```python
from build123d import *

# Parameters (mm, degrees)
SKETCH_1_R      = 77
SKETCH_1_R_2    = 75.75
EXTRUDE_1_DEPTH = 8
EXTRUDE_2_DEPTH = 3.9


with BuildPart() as part:
    # 草图1 → 凸台-拉伸1 (new body)
    with BuildSketch(Plane(origin=(0, 0, 0), x_dir=(1, 0, 0), z_dir=(0, 1, 0))):
        with Locations(Location((0, 0, 0), (0, 0, 270))):
            Circle(SKETCH_1_R)
        with Locations(Location((0, 0, 0), (0, 0, 270))):
            Circle(SKETCH_1_R_2, mode=Mode.SUBTRACT)
    extrude(amount=EXTRUDE_1_DEPTH)

    # 草图2 → 凸台-拉伸2 (add)
    with BuildSketch(Plane(origin=(0, 0, 0), x_dir=(1, 0, 0), z_dir=(0, 1, 0))):
        with BuildLine():
            Line((0, 75.75), (0, 74.85))
            ThreePointArc((0, 74.85), (27.43261682, 69.641754963), (51.047577251, 54.741824566))
            Line((51.047577251, 54.741824566), (51.661375775, 55.400042898))
            ThreePointArc((51.661375775, 55.400042898), (27.762467924, 70.479130775), (0, 75.75))
        make_face()
        with BuildLine():
            Line((55.400042898, -51.661375775), (54.741824566, -51.047577251))
            ThreePointArc((54.741824566, -51.047577251), (69.641754963, -27.43261682), (74.85, 0))
            Line((74.85, 0), (75.75, 0))
            ThreePointArc((75.75, 0), (70.479130775, -27.762467924), (55.400042898, -51.661375775))
        make_face()
        with BuildLine():
            Line((-51.661375775, -55.400042898), (-51.047577251, -54.741824566))
            ThreePointArc((-51.047577251, -54.741824566), (-27.43261682, -69.641754963), (0, -74.85))
            Line((0, -74.85), (0, -75.75))
            ThreePointArc((0, -75.75), (-27.762467924, -70.479130775), (-51.661375775, -55.400042898))
        make_face()
        with BuildLine():
            Line((-55.400042898, 51.661375775), (-54.741824566, 51.047577251))
            ThreePointArc((-54.741824566, 51.047577251), (-69.641754963, 27.43261682), (-74.85, 0))
            Line((-74.85, 0), (-75.75, 0))
            ThreePointArc((-75.75, 0), (-70.479130775, 27.762467924), (-55.400042898, 51.661375775))
        make_face()
    extrude(amount=EXTRUDE_2_DEPTH)


solid = part.part
```
Source: CAD feature listing. Evaluate the final solid. Frame: model axes, mm. A direction names the side the tool comes from. Coordinates: 2 decimals unless noted, no trailing zeros. Order: outer loops, then holes, each group sorted by start corner. A loop starts at its lowest first (then second) coordinate and runs counter-clockwise, first axis right, second up. Notation, with made-up numbers: M 36.5,-20 L 75.5,-20 A22 cw 75.5,9 Z; hole C -15,12 d2. An arc over 180 degrees is marked long. Write each question's results on one line, items separated by ' | '. Start each with the question number.
1) Section query B-B (x = -47.5). Return the cut outline in (y, z), plus the area to 3 significant figures.
2) Access query for faces 1 (the face through (-29.013, 4.833, 69.974)), 2 (the face through (-51, 8, 57)), 3 (the face through (27.066, 1.923, -69.785)). Directions: +Z, -Z, +X, -X, +Y, -Y. A direction counts if a zero-diameter tool reaches every point of the face in a straight line with its end or side. Return the directions, or none.
3) Line query: line 1 (Z direction, x = -1, y = 2.75); line 2 (X direction, y = 5, z = 0); line 3 (X direction, y = 7, z = -14). Output: solid intervals per line, ascending. Write a range as from..to.
4) Draft query along X for faces 4 (the face through (-75.17, 3.94, -16.69)), 5 (the face through (-17, 0, 74)), 6 (the face through (69.497, 1.923, 27.798)). Return one class per face: released by +X, released by -X, zero draft, split by the parting line, or undercut.
5) Section query C-C (z = -5). Return the cut outline in (x, y), plus the area to 3 significant figures.
6) Contact query for flat-ended pins moving along their axis: pin 1 Ø2 at (x, y) = (42.5, 5) entering from -Z; pin 2 Ø4 at (y, z) = (2, 4) entering from -X; pin 3 Ø3 at (x, y) = (-49, 4.5) entering from -Z; pin 4 Ø6.5 at (x, z) = (26, -66) entering from +Y. Output: stop coordinate, or through.
7) Section query A-A (y = 2.5). Return the cut outline in (x, z), plus the area to 3 significant figures.
Answers:
1) outline: M 0,-60.6 L 8,-60.6 L 8,-59.01 L 0,-59.01 Z; M 0,57.85 L 3.9,57.85 L 3.9,59.01 L 8,59.01 L 8,60.6 L 0,60.6 Z | area: 30.1 mm^2
2) face 1: +Y | face 2: +Z, -Z, +X, -X, +Y | face 3: +Y, -Y
3) line 1: z = -76.99..-75.74, 74.84..76.99 | line 2: x = -77..-75.75, 75.75..77 | line 3: x = -75.72..-74.45, 74.45..75.72
4) face 4: split by the parting line | face 5: zero draft | face 6: undercut
5) outline: M -76.84,0 L -74.68,0 L -74.68,3.9 L -75.58,3.9 L -75.58,8 L -76.84,8 Z; M 75.58,0 L 76.84,0 L 76.84,8 L 75.58,8 Z | area: 23.6 mm^2
6) pin 1: stops at z = -64.86 | pin 2: stops at x = -76.97 | pin 3: stops at z = -60.6 | pin 4: passes through
7) outline: C 0,0 d154; hole M -75.75,0 L -74.85,0 A74.85 ccw -54.74,-51.05 L -55.4,-51.66 A75.75 ccw 0,-75.75 L 0,-74.85 A74.85 ccw 51.05,-54.74 L 51.66,-55.4 A75.75 ccw 75.75,0 L 74.85,0 A74.85 ccw 54.74,51.05 L 55.4,51.66 A75.75 ccw 0,75.75 L 0,74.85 A74.85 ccw -51.05,54.74 L -51.66,55.4 A75.75 ccw Z | area: 803 mm^2
